Check sheet for the modelled part. Datum: model origin and axes. Units: mm. A direction names the side the tool comes from. Coordinates: 2 decimals unless noted, no trailing zeros. Write each loop counter-clockwise with the first axis right and the second up, starting at its lowest first coordinate (ties: lowest second). Pieces come first, ordered by that corner, then holes. Notation, with made-up numbers: M 77.25,6.25 L 129.25,6.25 A38 cw 129.25,44.25 Z; hole C 30,46 d7. An arc over 180 degrees is marked long. Answer as CSV lines item,"result". Start each with the question number.
Q1. Thickness scan on line 1 along Y through (x, z) = (2.25, -19.5) (3 decimals); line 2 along Z through (x, y) = (0.25, 3); line 3 along Y through (x, z) = (2.5, -12) (3 decimals). Record the ranges inside material, lowest first. Write a range as from..to.
Q2. Sectioned sample at C-C, the plane z = -2. Record the cut outline in (x, y) (3 decimals), then the cut area to 3 significant figures.
Q3. Depth check by flat-ended pin: pin 1 Ø3.5 at (y, z) = (-50.5, -10.5) entering from -X; pin 2 Ø2 at (x, z) = (4, -9.5) entering from -Y; pin 3 Ø0.8 at (x, z) = (4, 1.5) entering from +Y. Enter the tip coordinate at first touch or a pass-through.
Q4. Mould release check, pull along Z, two halves, no side actions. Record for faces 1 (the flat face through (3, 13.335, -7)), 2 (the flat face through (2.54, 42, 0)): pulls with the +Z half, pulls with the -Z half, needs draft (parallel to the pull), parting line crosses it, or undercut.
Q5. Sectioned sample at B-B, the plane y = 4. Record the cut outline in (x, z).
Q6. Sectioned sample at D-D, the plane z = -8.5. Record the cut outline in (x, y) (3 decimals).
Q7. Sectioned sample at A-A, the plane z = 3.5. Record the cut outline in (x, y) (3 decimals).
Q8. Access from +Z, -Z, +X, -X, +Y, -Y to the whole of each face (thin tool, end or side, straight path). Record for faces 3 (the flat face through (0, -50, 0)), 4 (the flat face through (2.54, -50, 0)), 5 (the flat face through (3, -1.905, -21)).
from build123d import *

# Parameters (mm, degrees)
F0_W     = 95.25
F0_H     = 46.99
F1_DEPTH = 2.54
F2_W     = 88.9
F2_H     = 46.99
F3_DEPTH = 2.54
F4_W     = 88.9
F4_H     = 46.99
F5_DEPTH = 1.27


with BuildPart() as f1:
    # F0 (on Right) → F1 (new body)
    with BuildSketch(Plane.YZ):
        with Locations((-3.81, -0.0466339131)):
            Rectangle(F0_W, F0_H)
        Polygon((-3.175, -2.9486645812), (-3.175, 2.1313354188), (13.335, 2.1313354188), (13.335, -16.9186645812), (5.715, -16.9186645812), (5.715, -19.4586645812), (-1.905, -19.4586645812), (-1.905, -21.9986645812), (-18.415, -21.9986645812), (-18.415, -5.4886645812), (-10.795, -5.4886645812), (-10.795, -2.9486645812), align=None, mode=Mode.SUBTRACT)
    extrude(amount=F1_DEPTH)

    # F2 (on face) → F3 (join)
    with BuildSketch(Plane.YZ.offset(2.54)):
        with Locations((-3.81, -0.0466339131)):
            Rectangle(F2_W, F2_H)
        Polygon((-18.415, -21.9986645812), (-18.415, -5.4886645812), (-10.795, -5.4886645812), (-10.795, -2.9486645812), (-3.175, -2.9486645812), (-3.175, 2.1313354188), (13.335, 2.1313354188), (13.335, -16.9186645812), (5.715, -16.9186645812), (5.715, -19.4586645812), (-1.905, -19.4586645812), (-1.905, -21.9986645812), align=None, mode=Mode.SUBTRACT)
    extrude(amount=F3_DEPTH)

    # F4 (on face) → F5 (join)
    with BuildSketch(Plane(origin=(0, 0, 0), x_dir=(0, -1, 0), z_dir=(-1, 0, 0))):
        with Locations((3.81, -0.0466339131)):
            Rectangle(F4_W, F4_H)
        Polygon((10.795, -2.9486645812), (10.795, -5.4886645812), (18.415, -5.4886645812), (18.415, -21.9986645812), (1.905, -21.9986645812), (1.905, -19.4586645812), (-5.715, -19.4586645812), (-5.715, -16.9186645812), (-13.335, -16.9186645812), (-13.335, 2.1313354188), (3.175, 2.1313354188), (3.175, -2.9486645812), align=None, mode=Mode.SUBTRACT)
        Polygon((18.415, -5.4886645812), (10.795, -5.4886645812), (10.795, -2.9486645812), (3.175, -2.9486645812), (3.175, 2.1313354188), (-13.335, 2.1313354188), (-13.335, -16.9186645812), (-5.715, -16.9186645812), (-5.715, -19.4586645812), (1.905, -19.4586645812), (1.905, -21.9986645812), (18.415, -21.9986645812), align=None)
    extrude(amount=F5_DEPTH)


solid = f1.part
Output:
1,line 1,"y = -51.435..-18.415, -1.905..43.815"
1,line 2,"z = -23.54..-19.46, 2.13..23.45"
1,line 3,"y = -51.435..-18.415, 13.335..43.815"
2,outline,"M -1.27,-48.26 L 0,-48.26 L 0,-51.435 L 2.54,-51.435 L 2.54,-48.26 L 5.08,-48.26 L 5.08,-3.175 L 0,-3.175 L 0,13.335 L 5.08,13.335 L 5.08,40.64 L 2.54,40.64 L 2.54,43.815 L 0,43.815 L 0,40.64 L -1.27,40.64 Z"
2,area,"497 mm^2"
3,pin 1,"stops at x = 0"
3,pin 2,"stops at y = -48.26"
3,pin 3,"stops at y = 40.64"
4,face 1,"undercut"
4,face 2,"needs draft"
5,outline,"M -1.27,-23.54 L 5.08,-23.54 L 5.08,-19.46 L 0,-19.46 L 0,2.13 L 5.08,2.13 L 5.08,23.45 L -1.27,23.45 Z"
6,outline,"M -1.27,-48.26 L 0,-48.26 L 0,-51.435 L 2.54,-51.435 L 2.54,-48.26 L 5.08,-48.26 L 5.08,-18.415 L 0,-18.415 L 0,13.335 L 5.08,13.335 L 5.08,40.64 L 2.54,40.64 L 2.54,43.815 L 0,43.815 L 0,40.64 L -1.27,40.64 Z"
7,outline,"M -1.27,-48.26 L 0,-48.26 L 0,-51.435 L 2.54,-51.435 L 2.54,-48.26 L 5.08,-48.26 L 5.08,40.64 L 2.54,40.64 L 2.54,43.815 L 0,43.815 L 0,40.64 L -1.27,40.64 Z"
8,face 3,"+Z, -Z, -X, -Y"
8,face 4,"+Z, -Z, +X, -Y"
8,face 5,"+X"
